For this review, take the finished solid that the model builds, in its own axes (mm). Round coordinates to 2 decimals unless told otherwise and drop trailing zeros. Order: outer loops, then holes, each group sorted by start corner. A loop starts at its lowest first (then second) coordinate and runs counter-clockwise, first axis right, second up. Notation, with made-up numbers: (6.25, 28.5) - (44.25, 28.5) arc R20 ccw to (44.25, 60.5) - close; hole circle Ø10 at (-23, 41.25). An arc over 180 degrees is marked (long way). One line per item, written item: value.
```python
from build123d import *

# Parameters (mm, degrees)
SKETCH_1_W                   = 12.7
SKETCH_1_H                   = 12.7
EXTRUDE_1_DEPTH              = 80.2
HOLE_WIZARD_M4_1_D           = 3.3
HOLE_WIZARD_M4_1_CSINK_D     = 3.35
HOLE_WIZARD_M4_1_CSINK_ANGLE = 90
HOLE_WIZARD_M5_1_D           = 4.2
HOLE_WIZARD_M5_1_CSINK_D     = 4.25
HOLE_WIZARD_M5_1_CSINK_ANGLE = 90


with BuildPart() as part:
    # 草圖1 → 填料-伸長1 (new body)
    with BuildSketch(Plane.XY):
        Rectangle(SKETCH_1_W, SKETCH_1_H)
    extrude(amount=EXTRUDE_1_DEPTH)

    # M4  螺絲攻的螺孔鑽1 (through all)
    with Locations(Plane(origin=(0, 6.35, 0), x_dir=(1, 0, 0), z_dir=(0, 1, 0))):
        with Locations((0, -60.1), (0, -75.1)):
            CounterSinkHole(HOLE_WIZARD_M4_1_D / 2, HOLE_WIZARD_M4_1_CSINK_D / 2, counter_sink_angle=HOLE_WIZARD_M4_1_CSINK_ANGLE)

    # M5  螺絲攻的螺孔鑽1 (through all)
    with Locations(Plane(origin=(0, 6.35, 0), x_dir=(1, 0, 0), z_dir=(0, 1, 0))):
        with Locations((0, -5.1), (0, -20.1)):
            CounterSinkHole(HOLE_WIZARD_M5_1_D / 2, HOLE_WIZARD_M5_1_CSINK_D / 2, counter_sink_angle=HOLE_WIZARD_M5_1_CSINK_ANGLE)


solid = part.part
```
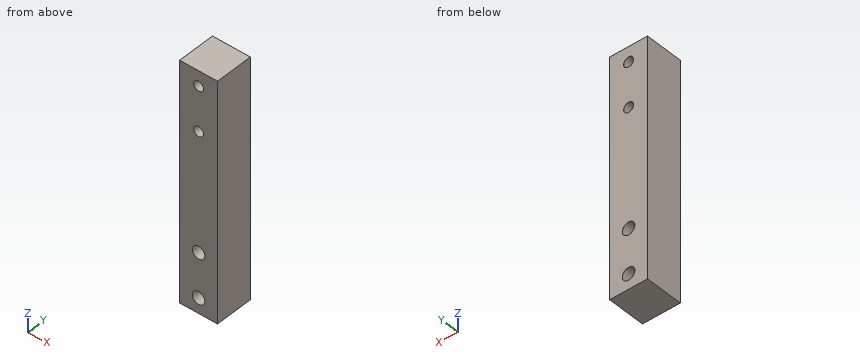
Item 1: Wall thickness on line 1 (Z direction, x = 0, y = 0); line 2 (Z direction, x = 0.5, y = 1); line 3 (X direction, y = 1, z = 60.1): over which ranges is each line inside the solid? List them lowest first.
Returned:
line 1: 0 to 3, 7.2 to 18, 22.2 to 58.45, 61.75 to 73.45, 76.75 to 80.2
line 2: 0 to 3.06, 7.14 to 18.06, 22.14 to 58.53, 61.67 to 73.53, 76.67 to 80.2
line 3: -6.35 to -1.65, 1.65 to 6.35
Item 2: For P1, Ø6.5, axis at x = 0, z = 5.1, coming from the +Y side; P2, Ø2.5, axis at x = 0, z = 75.1, coming from the -Y side, all flat-tipped, find the tip position at first contact; note any pin that passes through.
Returned:
P1: y = 6.35
P2: through
Item 3: Take a section at A-A (z = 60.1). Write out the cut boundary in (x, y) (3 decimals).
Returned:
outline: (-6.35, -6.35) - (-1.65, -6.35) - (-1.65, 6.325) - (-1.675, 6.35) - (-6.35, 6.35) - close; (1.65, -6.35) - (6.35, -6.35) - (6.35, 6.35) - (1.675, 6.35) - (1.65, 6.325) - close
Item 4: Take a section at B-B (y = -1.75). Write out the cut boundary in (x, z), plus the area to 3 significant figures.
Returned:
outline: (-6.35, 0) - (6.35, 0) - (6.35, 80.2) - (-6.35, 80.2) - close; hole circle Ø4.2 at (0, 5.1); hole circle Ø4.2 at (0, 20.1); hole circle Ø3.3 at (0, 60.1); hole circle Ø3.3 at (0, 75.1)
area: 974 mm^2
Item 5: Take a section at C-C (z = 20.1). Write out the cut boundary in (x, y) (3 decimals), plus the area to 3 significant figures.
Returned:
outline: (-6.35, -6.35) - (-2.1, -6.35) - (-2.1, 6.325) - (-2.125, 6.35) - (-6.35, 6.35) - close; (2.1, -6.35) - (6.35, -6.35) - (6.35, 6.35) - (2.125, 6.35) - (2.1, 6.325) - close
area: 108 mm^2
